Input: part model. Units: mm. Frame: model coordinates. Face numbers are marked on the shaded views. Round coordinates to 2 decimals unless told otherwise and drop trailing zeros. Loops run counter-clockwise (first coordinate to the right, second up) from the corner with the lowest first, then second, coordinate; pieces in that order, holes last. Notation, with made-up numbers: M 44.5,-26 L 72.5,-26 A23 ccw 72.5,3 Z; hole C 68.25,68.25 d6. An arc over 180 degrees is marked long. Put each result on its own line as item: value. Start each with the question number.
1) Section D-D on y = 11.5. Output: boundary loops of the cut face in (x, z).
2) Draft query along Y for the marked faces 1, 2 and 3. Return one class per face: +Y half, -Y half, draft (parallel to the pull), parting line (faces both ways), or undercut.
3) Pin query (flat end, axial travel): pin 1 (4.5 mm diameter, centred on x = 0, y = -10, fed in from +Z). Return the tip coordinate at first contact, or that it passes through.
4) Section C-C on z = 1.3. Output: boundary loops of the cut face in (x, y), plus the area to 3 significant figures.
5) Line query: probe 1 along Y at (x, z) = (0, 0.45); probe 2 along Y at (x, z) = (-1.25, 1); probe 3 along X at (y, z) = (-12, 0.7). Output: solid intervals per line, ascending.
6) Section B-B on x = -0.75. Output: boundary loops of the cut face in (y, z).
7) Section A-A on y = -10. Output: boundary loops of the cut face in (x, z), plus the area to 3 significant figures.
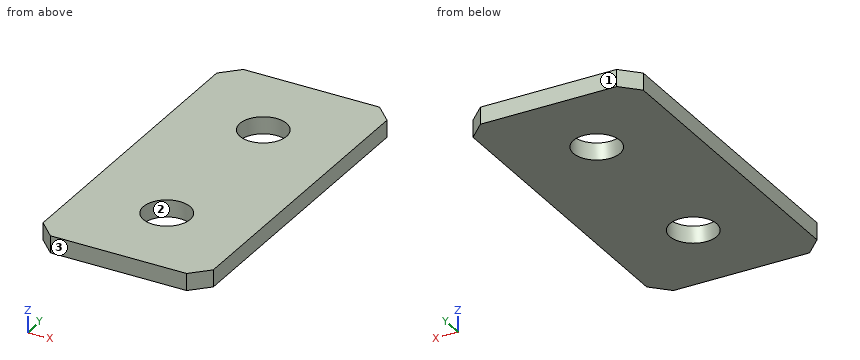
from build123d import *

# Parameters (mm, degrees)
SKETCH_1_W        = 20
SKETCH_1_H        = 40
EXTRUDE_1_DEPTH   = 2
CHAMFER_1_SIZE    = 2
HOLE_WIZARD_M51_D = 5.5


with BuildPart() as part:
    # Эскиз1 → Бобышка-Вытянуть1 (new body)
    with BuildSketch(Plane.XY):
        Rectangle(SKETCH_1_W, SKETCH_1_H)
    extrude(amount=EXTRUDE_1_DEPTH)

    # Фаска1
    chamfer_1_edges = [part.edges().sort_by_distance(p)[0] for p in [
        (10, -20, 1),
        (-10, -20, 1),
        (-10, 20, 1),
        (10, 20, 1),
    ]]
    chamfer(chamfer_1_edges, length=CHAMFER_1_SIZE)

    # Отверстие с зазором M51 (through all)
    with Locations(Plane.XY.offset(2)):
        with Locations((0, -30), (0, 30), (0, 10), (0, -10)):
            Hole(HOLE_WIZARD_M51_D / 2)


solid = part.part
Geometry results:
1. outline: M -10,0 L -2.3,0 L -2.3,2 L -10,2 Z; M 2.3,0 L 10,0 L 10,2 L 2.3,2 Z
2. face 1: +Y half
2. face 2: undercut
2. face 3: -Y half
3. pin 1: passes through
4. outline: M -10,-18 L -8,-20 L 8,-20 L 10,-18 L 10,18 L 8,20 L -8,20 L -10,18 Z; hole C 0,-10 d5.5; hole C 0,10 d5.5
4. area: 744 mm²
5. probe 1: y = -20 to -12.75, -7.25 to 7.25, 12.75 to 20
5. probe 2: y = -20 to -12.45, -7.55 to 7.55, 12.45 to 20
5. probe 3: x = -10 to -1.89, 1.89 to 10
6. outline: M -20,0 L -12.65,0 L -12.65,2 L -20,2 Z; M -7.35,0 L 7.35,0 L 7.35,2 L -7.35,2 Z; M 12.65,0 L 20,0 L 20,2 L 12.65,2 Z
7. outline: M -10,0 L -2.75,0 L -2.75,2 L -10,2 Z; M 2.75,0 L 10,0 L 10,2 L 2.75,2 Z
7. area: 29.0 mm²
